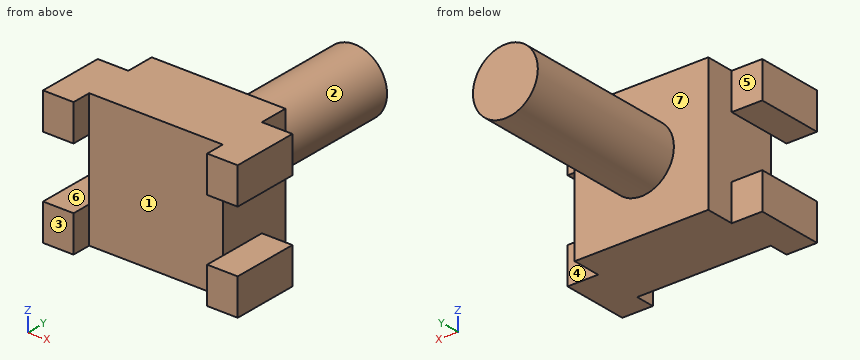
Autodesk Fusion 360 part; units mm, degrees
sketch "Sketch1" plane through (0, 0, 0) normal (0, 1, 0) x (1, 0, 0)
  line L0 (0, 0) -> (-7, 0)
  line L1 (-7, 0) -> (-7, -7)
  line L2 (-7, -7) -> (0, -7)
  line L3 (0, -7) -> (0, 0)
  dimension "d1" = 7
  dimension "d2" = 7
extrude "Extrude1" add sketch "Sketch1" along normal blind 4
sketch "Sketch2" plane through (0, 4, 0) normal (0, 1, 0) x (-1, 0, 0)
  line L0 (0, 7) -> (0, 0)
  line L1 (0, 0) -> (7, 0)
  line L2 (7, 0) -> (7, 7)
  line L3 (7, 7) -> (0, 7)
  line L4 (3.5, 7) -> (3.5, 0)
  line L5 (7, 3.5) -> (0, 3.5)
  circle A0 centre (3.5, 3.5) radius 1.7
  dimension "d5" = 3.4
extrude "Extrude2" add sketch "Sketch2" along normal blind 8.7 contours L4 L5 A0 | L4 L5 A0 | L4 L5 A0 | L4 L5 A0
ref_plane "WorkPlane1" through (-3.5, 0, 0) normal (1, 0, 0) x (0, 1, 0)
sketch "Sketch3" plane through (0, 0, 0) normal (1, 0, 0) x (0, 1, 0)
  line L0 (0, 7) -> (0, 0)
  line L1 (0, 0) -> (4, 0)
  line L2 (4, 0) -> (4, 7)
  line L3 (4, 7) -> (0, 7)
  line L4 (2.5, 0) -> (-1, 0)
  line L5 (-1, 0) -> (-1, 1.9)
  line L6 (-1, 1.9) -> (2.5, 1.9)
  line L7 (2.5, 1.9) -> (2.5, 0)
  line L8 (2.5, 7) -> (-1, 7)
  line L9 (-1, 7) -> (-1, 5.1)
  line L10 (-1, 5.1) -> (2.5, 5.1)
  line L11 (2.5, 5.1) -> (2.5, 7)
  line L12 (4, 7) -> (4, 0)
  dimension "d9" = 1.9
  dimension "d10" = 1.9
  dimension "d11" = 1.5
  dimension "d12" = 1.5
  dimension "d13" = 3.5
  dimension "d14" = 3.5
extrude "Extrude3" add sketch "Sketch3" along normal blind 1.6 contours L0 L3 L8 L10 L11 | L0 L8 L9 L10 | L0 L1 L4 L6 L7 | L0 L4 L5 L6
mirror "Mirror1" about plane through (-3.5, 0, 0) normal (1, 0, 0) of "Extrude3"
equation "d2 = d1"
equation "d10 = d9"
equation "d12 = d11"
equation "d14 = d13"
Geometry check sheet. Reference: the model listing, model coordinates, mm. Face numbers are marked on the shaded views. A direction names the side the tool comes from. Give positions to 0.01 mm unless a question says otherwise; leave off trailing zeros. Order: outer loops, then holes, each group sorted by start corner. A loop starts at its lowest first (then second) coordinate and runs counter-clockwise, first axis right, second up.
1. Gauge pin test, flat ends, axial feed: pin 1 Ø2 at (y, z) = (4, 5) entering from -X; pin 2 Ø3 at (y, z) = (8, 3) entering from -X; pin 3 Ø0.8 at (x, z) = (1, 1) entering from +Y; pin 4 Ø1 at (x, y) = (-1, 6) entering from -Z. Record the tip position at first contact, or that the pin passes through.
2. Section check A-A, the plane x = 0.5. Enter the section's corners in (y, z).
3. Section check C-C, the plane x = -3.5. Enter the section's corners in (y, z).
4. Access from +Z, -Z, +X, -X, +Y, -Y to the whole of each face (thin tool, end or side, straight path). Record for the marked faces 4, 5, 6 and 7.
5. Release check for a two-part mould opening along X. For the marked faces 1, 2 and 3 record: pulls with the +X half, pulls with the -X half, needs draft (parallel to the pull), parting line crosses it, or undercut.
6. Section check B-B, the plane z = 3.5. Enter the section's corners in (x, y), and give its area (3 significant figures).
7. Thickness scan on L1, parallel to Z at x = -8, y = 0.5; L2, parallel to Y at x = 0.5, z = 6.25; L3, parallel to Y at x = -3.75, z = 2.5. Record the ranges inside material, lowest first.
8. Section check D-D, the plane x = -6.5. Enter the section's corners in (y, z), and give its area (3 significant figures).
Values follow:
1. pin 1: stops at x = -7
1. pin 2: stops at x = -5.2
1. pin 3: stops at y = 2.5
1. pin 4: passes through
2. outline: (-1, 0) - (2.5, 0) - (2.5, 1.9) - (-1, 1.9) - close; (-1, 5.1) - (2.5, 5.1) - (2.5, 7) - (-1, 7) - close
3. outline: (0, 0) - (4, 0) - (4, 1.8) - (12.7, 1.8) - (12.7, 5.2) - (4, 5.2) - (4, 7) - (0, 7) - close
4. face 4: +Z, -Z, +X, +Y
4. face 5: +Z, -Z, -X, +Y
4. face 6: -X, +Y, -Y
4. face 7: +Y
5. face 1: undercut
5. face 2: parting line crosses it
5. face 3: needs draft
6. outline: (-7, 0) - (0, 0) - (0, 4) - (-1.8, 4) - (-1.8, 12.7) - (-5.2, 12.7) - (-5.2, 4) - (-7, 4) - close
6. area: 57.6 mm2
7. L1: z = 0 to 1.9, 5.1 to 7
7. L2: y = -1 to 2.5
7. L3: y = 0 to 12.7
8. outline: (0, 0) - (4, 0) - (4, 7) - (0, 7) - close
8. area: 28.0 mm2
